```python
from build123d import *

# Parameters (mm, degrees)
SALIENTE_EXTRUIR1_DEPTH           = 4.5
CORTAR_EXTRUIR1_DEPTH             = 3.2
DI_METRO_DE_TALADRO_1_0_1_1_D     = 1
DI_METRO_DE_TALADRO_1_0_1_1_DEPTH = 8
DI_METRO_DE_TALADRO_1_5_1_5_1_D   = 1.5


with BuildPart() as part:
    # Croquis1 → Saliente-Extruir1 (new body)
    with BuildSketch(Plane.XY.offset(4.5)):
        with BuildLine():
            Line((0, 8), (0, 0))
            Line((0, 0), (21.5, 0))
            ThreePointArc((21.5, 0), (18.55160392, 5.74555441), (12.5, 8))
            Line((12.5, 8), (0, 8))
        make_face()
    extrude(amount=-SALIENTE_EXTRUIR1_DEPTH)

    # Croquis2 → Cortar-Extruir1 (cut)
    with BuildSketch(Plane.XY.offset(4.5)):
        with BuildLine():
            Line((12.5, 7), (0, 7))
            Line((0, 7), (0, 0))
            Line((0, 0), (20.5, 0))
            ThreePointArc((20.5, 0), (17.892764807, 5.091731208), (12.5, 7))
        make_face()
    extrude(amount=-CORTAR_EXTRUIR1_DEPTH, mode=Mode.SUBTRACT)

    # Diámetro de taladro Ø1.0 (1)1
    with Locations(Plane(origin=(0, 8, 0), x_dir=(1, 0, 0), z_dir=(0, 1, 0))):
        with Locations((5, -2.65), (10, -2.65)):
            Hole(DI_METRO_DE_TALADRO_1_0_1_1_D / 2, depth=DI_METRO_DE_TALADRO_1_0_1_1_DEPTH)

    # Diámetro de taladro Ø1.5 (1.5)1 (through all)
    with Locations(Plane.XY.offset(1.3)):
        with Locations((10, 2.75), (5, 2.75)):
            Hole(DI_METRO_DE_TALADRO_1_5_1_5_1_D / 2)


solid = part.part
```
Model file for the job. Use its own axes, mm. A direction names the side the tool comes from. Give positions to 0.01 mm unless a question says otherwise; leave off trailing zeros. Loops run counter-clockwise (first coordinate to the right, second up) from the corner with the lowest first, then second, coordinate; pieces in that order, holes last. Notation, with made-up numbers: (3, 65) -> (24, 65) arc R24 ccw to (24, 103) -> close; hole circle Ø7 at (-30, 1). An arc over 180 degrees is marked (long way). Write each question's results on one line, items separated by ' | '.
(1) Probe line 1 along X through (y, z) = (2.5, 1); line 2 along Y through (x, z) = (10, 0.45); line 3 along Z through (x, y) = (10, 7.6). List the from-to ranges inside material, lowest first.
Geometry results:
line 1: x = 0 to 4.29, 5.71 to 9.29, 10.71 to 20.86 | line 2: y = 0 to 2, 3.5 to 8 | line 3: z = 0 to 2.15, 3.15 to 4.5
(2) Cut at C-C on z = 0.95. List the corners of the cut face in (x, y), and give its area (3 significant figures).
Geometry results:
outline: (0, 0) -> (21.5, 0) arc R8.93 ccw to (12.5, 8) -> (0, 8) -> close; hole circle Ø1.5 at (5, 2.75); hole circle Ø1.5 at (10, 2.75) | area: 152 mm²
(3) Flat gauge pins, fed straight in: pin 1 Ø1 at (x, z) = (16, 3) entering from -Y; pin 2 Ø2.5 at (x, y) = (10, 2.75) entering from +Z; pin 3 Ø1 at (y, z) = (3, 3) entering from -X. Where does each tip first touch, or does it go through?
Geometry results:
pin 1: stops at y = 6.06 | pin 2: stops at z = 1.3 | pin 3: stops at x = 19.28
(4) Cut at D-D on y = 7.5. List the corners of the cut face in (x, z).
Geometry results:
outline: (0, 0) -> (15.57, 0) -> (15.57, 4.5) -> (0, 4.5) -> close; hole circle Ø1 at (5, 2.65); hole circle Ø1 at (10, 2.65)
(5) Tool access for faces 4 (the flat face through (6, 7, 3)), 5 (the cylindrical face through (10.75, 2.78, 0.64)): list every direction of +Z, -Z, +X, -X, +Y, -Y with a clear straight run to the whole face (end or side of a thin tool).
Geometry results:
face 4: +Z, -X, -Y | face 5: +Z, -Z
(6) Cut at B-B on x = 10. List the corners of the cut face in (y, z).
Geometry results:
outline: (0, 0) -> (2, 0) -> (2, 1.3) -> (0, 1.3) -> close; (3.5, 0) -> (8, 0) -> (8, 2.15) -> (7, 2.15) -> (7, 1.3) -> (3.5, 1.3) -> close; (7, 3.15) -> (8, 3.15) -> (8, 4.5) -> (7, 4.5) -> close
(7) Cut at A-A on z = 2.35. List the corners of the cut face in (x, y), and give its area (3 significant figures).
Geometry results:
outline: (0, 7) -> (4.6, 7) -> (4.6, 8) -> (0, 8) -> close; (5.4, 7) -> (9.6, 7) -> (9.6, 8) -> (5.4, 8) -> close; (10.4, 7) -> (12.5, 7) arc R7.74 cw to (20.5, 0) -> (21.5, 0) arc R8.93 ccw to (12.5, 8) -> (10.4, 8) -> close | area: 22.7 mm²
(8) Pull direction Z, two halves, no side cores. Call faces 1 (the flat face through (10, 4, 1.3)), 2 (the cylindrical face through (17.95, 5.04, 2.92)), 3 (the cylindrical face through (10.4, 7.49, 2.95)): released by +Z, released by -Z, zero draft, split by the parting line, or undercut.
Geometry results:
face 1: released by +Z | face 2: zero draft | face 3: undercut
